CAD build for the part. Positions are in the model's coordinates, mm. A direction names the side the tool comes from. Round coordinates to 2 decimals unless told otherwise and drop trailing zeros. Order: outer loops, then holes, each group sorted by start corner. A loop starts at its lowest first (then second) coordinate and runs counter-clockwise, first axis right, second up. Notation, with made-up numbers: (13, 35) - (39, 35) arc R14 ccw to (39, 46) - close; hole circle Ø6 at (33, 23.5). An arc over 180 degrees is marked (long way). Use one line per item in the form item = value. Start each with the question number.
from build123d import *

# Parameters (mm, degrees)
SKETCH2_W                = 70
SKETCH2_H                = 10
SKETCH3_R                = 25
CUT_EXTRUDE1_DEPTH       = 91
SKETCH4_R                = 25
BOSS_EXTRUDE1_DEPTH      = 10
BOSS_EXTRUDE1_DEPTH_BACK = 100


with BuildPart() as part:
    # Sweep1: sweep along a path in Sketch1
    with BuildLine(Plane.XY) as sweep1_path:
        Line((48.354821102, -220), (48.354821102, -10))
        ThreePointArc((48.354821102, -10), (45.425888913, -2.928932188), (38.354821102, 0))
        Line((38.354821102, 0), (-21.645178898, 0))
        ThreePointArc((-21.645178898, 0), (-28.71624671, -2.928932188), (-31.645178898, -10))
        Line((-31.645178898, -10), (-31.645178898, -220))
    # Sketch2 → Sweep1 (sweep)
    with BuildSketch(Plane(origin=(0, 0, 0), x_dir=(0, 0, -1), z_dir=(1, 0, 0))):
        Rectangle(SKETCH2_W, SKETCH2_H)
    sweep(path=sweep1_path.line)

    # Sketch3 → Cut-Extrude1 (cut, through all)
    with BuildSketch(Plane(origin=(53.354821102, 0, 0), x_dir=(0, 0, -1), z_dir=(1, 0, 0))):
        with Locations((0, -175)):
            Circle(SKETCH3_R)
    extrude(amount=-CUT_EXTRUDE1_DEPTH, mode=Mode.SUBTRACT)

    # Sketch4 → Boss-Extrude1 (add, two sides)
    with BuildSketch(Plane(origin=(53.354821102, 0, 0), x_dir=(0, 0, -1), z_dir=(1, 0, 0))) as boss_extrude1_sk:
        with Locations((0, -175)):
            Circle(SKETCH4_R)
    extrude(amount=BOSS_EXTRUDE1_DEPTH)
    extrude(boss_extrude1_sk.sketch, amount=-BOSS_EXTRUDE1_DEPTH_BACK)


solid = part.part
(1) Mould opens along Y. For faces 5 (the flat face through (43.355, -114, 0)), 6 (the cylindrical face through (49.077, 0.489, 0.49)), 7 (the flat face through (-32, -220, 0)) say: pulls with the +Y half, pulls with the -Y half, needs draft (parallel to the pull), parting line crosses it, or undercut.
(2) Slice it at C-C (x = 26). Give the cut face in (y, z).
(3) Flat gauge pins, fed straight in: P1, Ø1, axis at y = -140, z = 26.5, coming from the -X side; P2, Ø2, axis at x = -25.5, z = 24.5, coming from the +Y side; P3, Ø12, axis at y = -138.5, z = -7.5, coming from the +X side. Where does each tip first touch, or does it go through?
(4) Which spindle directions (+Z, -Z, +X, -X, +Y, -Y) get a long thin tool onto all of the face, cutting with end or side? Do faces 1 (the cylindrical face through (8.845, -150.213, 3.255)), 2 (the flat face through (8, -5, 0)), 3 (the cylindrical face through (-41.575, -150.213, 3.255)), 4 (the cylindrical face through (58.285, -150.213, 3.255)). Say none if no direction does.
(5) Slice it at B-B (z = 20). Give the cut face in (x, y).
(6) Slice it at D-D (y = -175). Give the cut face in (x, z), and give its area (3 significant figures).
(7) Wall check: line 1 (X direction, y = -60, z = 4.5); line 2 (Y direction, x = 26, z = 15.5); line 3 (Y direction, x = 14, z = 22.5). Give the ranges that are in metal, low to high. Write a range as [from, to].
(8) Slice it at A-A (y = -35). Give the cut face in (x, z).
Results list:
q1.face_5 = undercut
q1.face_6 = pulls with the +Y half
q1.face_7 = pulls with the -Y half
q2.outline = circle Ø50 at (-175, 0); (-5, -35) - (5, -35) - (5, 35) - (-5, 35) - close
q3.P1 = -36.65
q3.P2 = 4.73
q3.P3 = 53.35
q4.face_1 = none
q4.face_2 = +Z, -Z
q4.face_3 = -X
q4.face_4 = +X
q5.outline = (-46.65, -190) - (-36.65, -190) - (-36.65, -220) - (-26.65, -220) - (-26.65, -190) - (43.35, -190) - (43.35, -220) - (53.35, -220) - (53.35, -190) - (63.35, -190) - (63.35, -160) - (53.35, -160) - (53.35, -10) arc R15 ccw to (38.35, 5) - (-21.65, 5) arc R15 ccw to (-36.65, -10) - (-36.65, -160) - (-46.65, -160) - close; hole (-26.65, -160) - (43.35, -160) - (43.35, -10) arc R5 ccw to (38.35, -5) - (-21.65, -5) arc R5 ccw to (-26.65, -10) - close
q6.outline = (-46.65, -25) - (-36.65, -25) - (-36.65, -35) - (-26.65, -35) - (-26.65, -25) - (43.35, -25) - (43.35, -35) - (53.35, -35) - (53.35, -25) - (63.35, -25) - (63.35, 25) - (53.35, 25) - (53.35, 35) - (43.35, 35) - (43.35, 25) - (-26.65, 25) - (-26.65, 35) - (-36.65, 35) - (-36.65, 25) - (-46.65, 25) - close
q6.area = 5,900 mm²
q7.line_1 = [-36.65, -26.65], [43.35, 53.35]
q7.line_2 = [-194.62, -155.38], [-5, 5]
q7.line_3 = [-185.9, -164.1], [-5, 5]
q8.outline = (-36.65, -35) - (-26.65, -35) - (-26.65, 35) - (-36.65, 35) - close; (43.35, -35) - (53.35, -35) - (53.35, 35) - (43.35, 35) - close
